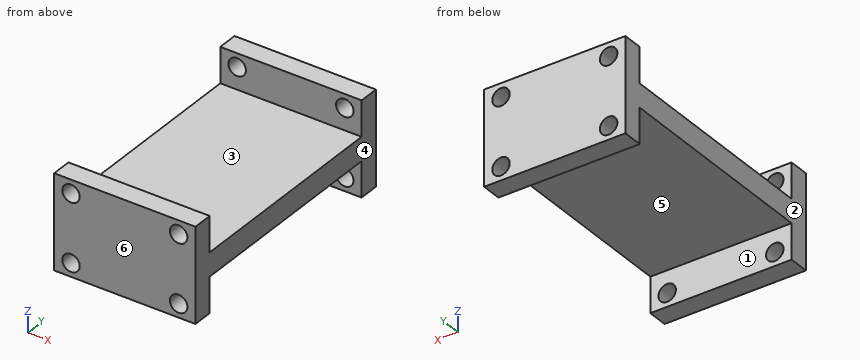
from build123d import *

# Parameters (mm, degrees)
SKETCH3_W           = 21
SKETCH3_H           = 14
SKETCH3_R           = 1.3
BOSS_EXTRUDE1_DEPTH = 3
SKETCH4_W           = 21
SKETCH4_H           = 3.5
BOSS_EXTRUDE2_DEPTH = 32
SKETCH5_W           = 21
SKETCH5_H           = 14
SKETCH5_R           = 1.3
BOSS_EXTRUDE3_DEPTH = 3


with BuildPart() as part:
    # Sketch3 → Boss-Extrude1 (new body)
    with BuildSketch(Plane(origin=(0, 0, 0), x_dir=(1, 0, 0), z_dir=(0, 1, 0))):
        Rectangle(SKETCH3_W, SKETCH3_H)
        with Locations(Location((-8, -5, 0), (0, 0, 270))):
            Circle(SKETCH3_R, mode=Mode.SUBTRACT)
        with Locations(Location((8, -5, 0), (0, 0, 270))):
            Circle(SKETCH3_R, mode=Mode.SUBTRACT)
        with Locations(Location((8, 5, 0), (0, 0, 90))):
            Circle(SKETCH3_R, mode=Mode.SUBTRACT)
        with Locations(Location((-8, 5, 0), (0, 0, 90))):
            Circle(SKETCH3_R, mode=Mode.SUBTRACT)
    extrude(amount=BOSS_EXTRUDE1_DEPTH)

    # Sketch4 → Boss-Extrude2 (add)
    with BuildSketch(Plane(origin=(0, 3, 0), x_dir=(1, 0, 0), z_dir=(0, 1, 0))):
        Rectangle(SKETCH4_W, SKETCH4_H)
    extrude(amount=BOSS_EXTRUDE2_DEPTH)

    # Sketch5 → Boss-Extrude3 (add)
    with BuildSketch(Plane(origin=(0, 35, 0), x_dir=(1, 0, 0), z_dir=(0, 1, 0))):
        Rectangle(SKETCH5_W, SKETCH5_H)
        with Locations(Location((-8, -5, 0), (0, 0, 270))):
            Circle(SKETCH5_R, mode=Mode.SUBTRACT)
        with Locations(Location((-8, 5, 0), (0, 0, 90))):
            Circle(SKETCH5_R, mode=Mode.SUBTRACT)
        with Locations(Location((8, 5, 0), (0, 0, 90))):
            Circle(SKETCH5_R, mode=Mode.SUBTRACT)
        with Locations(Location((8, -5, 0), (0, 0, 270))):
            Circle(SKETCH5_R, mode=Mode.SUBTRACT)
    extrude(amount=BOSS_EXTRUDE3_DEPTH)


solid = part.part
Could you check a few things on this model? Use its own coordinates, in mm. Face numbers are marked on the shaded views. A direction names the side the tool comes from. Round coordinates to 2 decimals unless told otherwise and drop trailing zeros. Order: outer loops, then holes, each group sorted by start corner. A loop starts at its lowest first (then second) coordinate and runs counter-clockwise, first axis right, second up.
Q1. Which directions (+Z, -Z, +X, -X, +Y, -Y) give clear straight access to the entire face, cutting with the end or side of a thin tool? Please do the marked faces 1, 2 and 3.
Geometry says:
face 1: -Z, +X, -X
face 2: +Z, -Z, -X, +Y, -Y
face 3: +Z, +X, -X
Q2. Please list where these lines run through material, in increasing order: probe 1 along X at (y, z) = (36.55, -5); probe 2 along Y at (x, z) = (-2, 6.75); probe 3 along X at (y, z) = (2, -4.25).
Geometry says:
probe 1: x = -10.5 to -9.3, -6.7 to 6.7, 9.3 to 10.5
probe 2: y = 0 to 3, 35 to 38
probe 3: x = -10.5 to -9.06, -6.94 to 6.94, 9.06 to 10.5
Q3. Imagine slicing it at C-C, the plane z = 3.25. List the corners of the cut face in (x, y) for me, then the cut area to 3 significant figures.
Geometry says:
outline: (-10.5, 0) - (10.5, 0) - (10.5, 3) - (-10.5, 3) - close; (-10.5, 35) - (10.5, 35) - (10.5, 38) - (-10.5, 38) - close
area: 126 mm2
Q4. Imagine slicing it at A-A, the plane x = -8.5. List the corners of the cut face in (y, z) for me, then the cut area to 3 significant figures.
Geometry says:
outline: (0, -7) - (3, -7) - (3, -6.2) - (0, -6.2) - close; (0, -3.8) - (3, -3.8) - (3, -1.75) - (35, -1.75) - (35, -3.8) - (38, -3.8) - (38, 3.8) - (35, 3.8) - (35, 1.75) - (3, 1.75) - (3, 3.8) - (0, 3.8) - close; (0, 6.2) - (3, 6.2) - (3, 7) - (0, 7) - close; (35, -7) - (38, -7) - (38, -6.2) - (35, -6.2) - close; (35, 6.2) - (38, 6.2) - (38, 7) - (35, 7) - close
area: 167 mm2
Q5. I'm going to push flat-ended pins straight in: P1, Ø2.5, axis at x = -1, z = -5, coming from the -Y side; P2, Ø12, axis at x = -4, y = 10, coming from the +Z side; P3, Ø6.5, axis at x = -3, y = 18.5, coming from the -Z side. Where does each tip first touch, or does it pass through?
Geometry says:
P1: stops at y = 0
P2: stops at z = 1.75
P3: stops at z = -1.75
Q6. Thinking about a two-plate mould opening in Y: for the marked faces 4, 5 and 6, which applies, released by +Y, released by -Y, zero draft, split by the parting line, or undercut?
Geometry says:
face 4: zero draft
face 5: undercut
face 6: released by -Y
Q7. Imagine slicing it at B-B, the plane z = -4.5. List the corners of the cut face in (x, y) for me.
Geometry says:
outline: (-10.5, 0) - (-9.2, 0) - (-9.2, 3) - (-10.5, 3) - close; (-10.5, 35) - (-9.2, 35) - (-9.2, 38) - (-10.5, 38) - close; (-6.8, 0) - (6.8, 0) - (6.8, 3) - (-6.8, 3) - close; (-6.8, 35) - (6.8, 35) - (6.8, 38) - (-6.8, 38) - close; (9.2, 0) - (10.5, 0) - (10.5, 3) - (9.2, 3) - close; (9.2, 35) - (10.5, 35) - (10.5, 38) - (9.2, 38) - close
Q8. Imagine slicing it at D-D, the plane x = -2.5. List the corners of the cut face in (y, z) for me, then the cut area to 3 significant figures.
Geometry says:
outline: (0, -7) - (3, -7) - (3, -1.75) - (35, -1.75) - (35, -7) - (38, -7) - (38, 7) - (35, 7) - (35, 1.75) - (3, 1.75) - (3, 7) - (0, 7) - close
area: 196 mm2
